The model under review builds one solid part; all positions refer to its coordinate system, in mm. Face numbers are marked on the shaded views. A direction names the side the tool comes from. Give positions to 0.01 mm unless a question says otherwise; leave off trailing zeros. Order: outer loops, then holes, each group sorted by start corner. A loop starts at its lowest first (then second) coordinate and runs counter-clockwise, first axis right, second up.
```python
from build123d import *

# Parameters (mm, degrees)
F0_R     = 127
F1_DEPTH = 19.05
F2_R     = 12.7
F3_DEPTH = 254
F4_R     = 10.755444
F5_DEPTH = 50.8


with BuildPart() as f1:
    # F0 (on Top) → F1 (new body)
    with BuildSketch(Plane.XY):
        Circle(F0_R)
    extrude(amount=F1_DEPTH)

    # F2 (on face) → F3 (join)
    with BuildSketch(Plane(origin=(0, 0, 0), x_dir=(1, 0, 0), z_dir=(0, 0, -1))):
        Circle(F2_R)
    extrude(amount=F3_DEPTH)

    # F4 (on face) → F5 (cut)
    with BuildSketch(Plane(origin=(0, 0, -254), x_dir=(1, 0, 0), z_dir=(0, 0, -1))):
        Circle(F4_R)
    extrude(amount=-F5_DEPTH, mode=Mode.SUBTRACT)


solid = f1.part
```
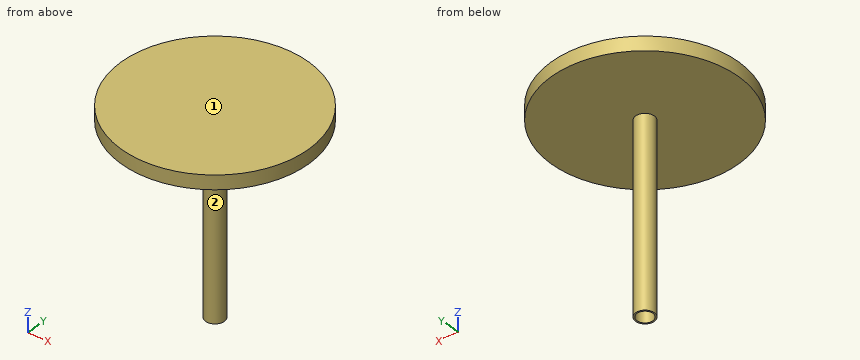
1. Take a section at A-A (y = 0). Write out the cut boundary in (x, z), and give its area (3 significant figures).
2. For the marked faces 1 and 2, list the 3-axis set-ups (+Z, -Z, +X, -X, +Y, -Y) from which the entire face can be reached by the end or side of a thin tool; tool diameter is ignored.
3. Take a section at C-C (z = -234). Write out the cut boundary in (x, y).
4. To check wall thickness, follow line 1 (Y direction, x = 0, z = -225.5); line 2 (Z direction, x = 112.5, y = -28.5). State the ranges of each line that lie inside material, in increasing order.
5. Insertion check: pin 1 (3 mm diameter, centred on x = -4.5, y = -21.5, fed in from -Z); pin 2 (2 mm diameter, centred on y = 1, z = -182.5, fed in from +X). Each pin has a flat end and moves straight along its axis. Give the tip position at first contact, or say it passes through.
6. Take a section at D-D (z = -132.5). Write out the cut boundary in (x, y).
Answer:
1. outline: (-127, 0) - (-12.7, 0) - (-12.7, -254) - (-10.76, -254) - (-10.76, -203.2) - (10.76, -203.2) - (10.76, -254) - (12.7, -254) - (12.7, 0) - (127, 0) - (127, 19.05) - (-127, 19.05) - close
1. area: 10,200 mm2
2. face 1: +Z, +X, -X, +Y, -Y
2. face 2: -Z
3. outline: circle Ø25.4 at (0, 0); hole circle Ø21.51 at (0, 0)
4. line 1: y = -12.7 to -10.76, 10.76 to 12.7
4. line 2: z = 0 to 19.05
5. pin 1: stops at z = 0
5. pin 2: stops at x = 12.7
6. outline: circle Ø25.4 at (0, 0)
